For this review, take the finished solid that the model builds, in its own axes (mm). A direction names the side the tool comes from. Round coordinates to 2 decimals unless told otherwise and drop trailing zeros. Write each loop counter-clockwise with the first axis right and the second up, starting at its lowest first coordinate (ties: lowest second). Pieces come first, ordered by that corner, then holes. Notation, with made-up numbers: M -9.5,60 L 12.5,60 A25 cw 12.5,89 Z; hole C 38.25,-28 d1. An arc over 180 degrees is marked long. Use one line per item in the form item = value. Start each with the question number.
Item 1: Add section A-A (y = -1.85). State the section outline as (x, z) points.
Item 2: Add section B-B (x = -20). State the section outline as (y, z) points.
Item 3: Draft analysis for pull direction Z (two halves, no side actions). For faces 1 (the cylindrical face through (-35.147, -1.479, -51.337)), 2 (the flat face through (-1, -3, -53)), 3 (the flat face through (27.3, -1.48, -64.86)), state which applies: released by +Z, released by -Z, zero draft, split by the parting line, or undercut.
Item 4: For faces 4 (the flat face through (-7, -1, -56.655)), 5 (the flat face through (-1, 0, -53)), 6 (the flat face through (-6, -1, -46.457)), list the 3-axis set-ups (+Z, -Z, +X, -X, +Y, -Y) from which the entire face can be reached by the end or side of a thin tool; tool diameter is ignored.
Item 5: For P1, Ø1.5, axis at x = -12, y = -2, coming from the +Z side, flat-tipped, find the tip position at first contact; note if it passes through.
Item 6: Add section C-C (z = -54.5). State the section outline as (x, y) points, and give its area (3 significant figures).
Item 7: For line 1 (X direction, y = -1.9, z = -57.75); line 2 (Z direction, x = -19, y = -0.3); line 3 (X direction, y = -2.75, z = -59), list the stretches that pass through material, from the lowest coordinate up. Write a range as [from, to].
from build123d import *

# Parameters (mm, degrees)
F1_DEPTH = 3
F3_DEPTH = 25


# Not quite as in the source:
# - a feature names something its author has since deleted; it is built from what else it names


with BuildPart() as f1:
    # F0 (on Front) → F1 (new body)
    with BuildSketch(Plane.XZ):
        with BuildLine():
            Line((-24.6447846293, -46.4568324387), (-24.6447846293, -56.6546805203))
            Line((-24.6447846293, -56.6546805203), (-23.8253123528, -56.6546805203))
            ThreePointArc((-23.8253123528, -56.6546805203), (-22.130084006, -54.3516793641), (-21.5297268649, -51.5557564795))
            ThreePointArc((-21.5297268649, -51.5557564795), (-22.130084006, -48.7598335949), (-23.8253123528, -46.4568324387))
            Line((-23.8253123528, -46.4568324387), (-24.6447846293, -46.4568324387))
        make_face()
        with BuildLine():
            Line((-23.8253123528, -56.6546805203), (-24.6447846293, -56.6546805203))
            Line((-24.6447846293, -56.6546805203), (-24.6447846293, -46.4568324387))
            Line((-24.6447846293, -46.4568324387), (-23.8253123528, -46.4568324387))
            ThreePointArc((-23.8253123528, -46.4568324387), (-35.1509748081, -51.5557564795), (-23.8253123528, -56.6546805203))
        make_face()
        with BuildLine():
            ThreePointArc((-21.5297268649, -51.5557564795), (-22.130084006, -54.3516793641), (-23.8253123528, -56.6546805203))
            Line((-23.8253123528, -56.6546805203), (11.1679025889, -56.6546805203))
            ThreePointArc((11.1679025889, -56.6546805203), (8.8185102803, -51.5557564795), (11.1679025889, -46.4568324387))
            Line((11.1679025889, -46.4568324387), (-23.8253123528, -46.4568324387))
            ThreePointArc((-23.8253123528, -46.4568324387), (-22.130084006, -48.7598335949), (-21.5297268649, -51.5557564795))
        make_face()
        with BuildLine():
            ThreePointArc((11.1679025889, -46.4568324387), (8.8185102803, -51.5557564795), (11.1679025889, -56.6546805203))
            Line((11.1679025889, -56.6546805203), (11.8974819779, -56.6546805203))
            Line((11.8974819779, -56.6546805203), (11.8974819779, -46.4568324387))
            Line((11.8974819779, -46.4568324387), (11.1679025889, -46.4568324387))
        make_face()
        with BuildLine():
            Line((11.8974819779, -56.6546805203), (11.1679025889, -56.6546805203))
            ThreePointArc((11.1679025889, -56.6546805203), (14.8431416467, -58.2287078356), (18.7610955863, -57.4321018799))
            ThreePointArc((18.7610955863, -57.4321018799), (20.0078661899, -55.0037023767), (22.0355331957, -53.1761007794))
            ThreePointArc((22.0355331957, -53.1761007794), (22.1843328788, -52.371994204), (22.234179719, -51.5557564795))
            ThreePointArc((22.234179719, -51.5557564795), (18.3334195709, -45.4635172382), (11.1679025889, -46.4568324387))
            Line((11.1679025889, -46.4568324387), (11.8974819779, -46.4568324387))
            Line((11.8974819779, -46.4568324387), (11.8974819779, -56.6546805203))
        make_face()
        with BuildLine():
            ThreePointArc((22.0355331957, -53.1761007794), (20.0078661899, -55.0037023767), (18.7610955863, -57.4321018799))
            ThreePointArc((18.7610955863, -57.4321018799), (20.8427791516, -55.6460589781), (22.0355331957, -53.1761007794))
        make_face()
        with BuildLine():
            ThreePointArc((22.0355331957, -53.1761007794), (20.8427791516, -55.6460589781), (18.7610955863, -57.4321018799))
            ThreePointArc((18.7610955863, -57.4321018799), (24.8985692809, -67.0974714468), (33.5650116518, -59.615444392))
            ThreePointArc((33.5650116518, -59.615444392), (29.6898526428, -53.0125279979), (22.0355331957, -53.1761007794))
        make_face()
    extrude(amount=F1_DEPTH)

    # F2 (on face) → F3 (cut)
    with BuildSketch(Plane(origin=(0, 0, 0), x_dir=(-1, 0, 0), z_dir=(0, 1, 0))):
        with BuildLine():
            ThreePointArc((-26.7674391798, -62.7047392847), (-28.3016132323, -61.8158013566), (-29.1220744495, -60.2439412946))
            Line((-29.1220744495, -60.2439412946), (-33.4160842435, -61.108925342))
            ThreePointArc((-33.4160842435, -61.108925342), (-31.4664434529, -64.8440957921), (-27.8208252933, -66.9564560213))
            Line((-27.8208252933, -66.9564560213), (-26.7674391798, -62.7047392847))
        make_face()
        with BuildLine():
            ThreePointArc((-27.8208252933, -66.9564560213), (-31.4664434529, -64.8440957921), (-33.4160842435, -61.108925342))
            Line((-33.4160842435, -61.108925342), (-39.6901629865, -62.3727738857))
            Line((-39.6901629865, -62.3727738857), (-29.0901046246, -72.0795691013))
            Line((-29.0901046246, -72.0795691013), (-27.8208252933, -66.9564560213))
        make_face()
        with BuildLine():
            Line((-26.0020494461, -59.615444392), (-29.1220744495, -60.2439412946))
            ThreePointArc((-29.1220744495, -60.2439412946), (-28.3016132323, -61.8158013566), (-26.7674391798, -62.7047392847))
            Line((-26.7674391798, -62.7047392847), (-26.0020494461, -59.615444392))
        make_face()
        with BuildLine():
            ThreePointArc((-26.7674391798, -62.7047392847), (-24.0407284287, -62.1219926651), (-22.8193517887, -59.615444392))
            ThreePointArc((-22.8193517887, -59.615444392), (-26.3178564355, -56.4484536556), (-29.1220744495, -60.2439412946))
            Line((-29.1220744495, -60.2439412946), (-26.0020494461, -59.615444392))
            Line((-26.0020494461, -59.615444392), (-26.7674391798, -62.7047392847))
        make_face()
    extrude(amount=-F3_DEPTH, mode=Mode.SUBTRACT)


solid = f1.part
Calculated:
q1.outline = M -23.83,-56.65 L 11.17,-56.65 A6.71 ccw 18.76,-57.43 A7.56 ccw 27.82,-66.96 L 26.77,-62.7 A3.18 cw long 29.12,-60.24 L 33.42,-61.11 A7.56 ccw 22.04,-53.18 A6.71 ccw 11.17,-46.46 L -23.83,-46.46 A6.81 ccw long Z
q2.outline = M -3,-56.65 L 0,-56.65 L 0,-46.46 L -3,-46.46 Z
q3.face_1 = split by the parting line
q3.face_2 = zero draft
q3.face_3 = undercut
q4.face_4 = -Z, +Y, -Y
q4.face_5 = +Z, -Z, +X, -X, +Y
q4.face_6 = +Z, +Y, -Y
q5.P1 = -46.46
q6.outline = M -34.48,-3 L 31.57,-3 L 31.57,0 L -34.48,0 Z
q6.area = 198 mm^2
q7.line_1 = [-31.17, -25.51], [12.95, 18.1], [18.67, 23.42], [28.58, 33.33]
q7.line_2 = [-56.65, -46.46]
q7.line_3 = [18.46, 22.88], [29.12, 33.54]
